```python
from build123d import *

# Parameters (mm, degrees)
SKETCH1_W               = 50.8
SKETCH1_H               = 25.4
BOSS_EXTRUDE1_DEPTH     = 3.999992
CUT_EXTRUDE1_DEPTH      = 57.936806514
CUT_EXTRUDE1_DEPTH_BACK = 57.936806514
SKETCH2_W               = 13.999972
SKETCH2_H               = 13.999972
SKETCH3_W               = 4.998974
SKETCH3_H               = 1.307084
CUT_EXTRUDE2_DEPTH      = 2.500122
BOSS_EXTRUDE2_DEPTH     = 50.8
FILLET1_R               = 1.5875


with BuildPart() as part:
    # Sketch1 → Boss-Extrude1 (new body)
    with BuildSketch(Plane(origin=(0, 0, 0), x_dir=(1, 0, 0), z_dir=(0, 1, 0))):
        with Locations((25.4, 12.7)):
            Rectangle(SKETCH1_W, SKETCH1_H)
    extrude(amount=BOSS_EXTRUDE1_DEPTH)

    # Sketch2 → Cut-Extrude1 (cut, two sides: drawn at the far end of the back side and taken through both)
    with BuildSketch(Plane(origin=(0, 3.999992, 0), x_dir=(1, 0, 0), z_dir=(0, 1, 0)).offset(-CUT_EXTRUDE1_DEPTH_BACK)):
        with Locations((15.875508, 12.7)):
            Rectangle(SKETCH2_W, SKETCH2_H)
        with Locations((34.924492, 12.7)):
            Rectangle(SKETCH2_W, SKETCH2_H)
    extrude(amount=CUT_EXTRUDE1_DEPTH + CUT_EXTRUDE1_DEPTH_BACK, mode=Mode.SUBTRACT)

    # Sketch3 → Cut-Extrude2 (cut)
    with BuildSketch(Plane(origin=(0, 3.999992, 0), x_dir=(1, 0, 0), z_dir=(0, 1, 0))):
        with Locations((15.875508, 20.353528)):
            Rectangle(SKETCH3_W, SKETCH3_H)
        with Locations((34.924492, 20.353528)):
            Rectangle(SKETCH3_W, SKETCH3_H)
        with Locations((34.924492, 5.046472)):
            Rectangle(SKETCH3_W, SKETCH3_H)
        with Locations((15.875508, 5.046472)):
            Rectangle(SKETCH3_W, SKETCH3_H)
    extrude(amount=-CUT_EXTRUDE2_DEPTH, mode=Mode.SUBTRACT)

    # Sketch5 → Boss-Extrude2 (add)
    with BuildSketch(Plane.ZY):
        Polygon((0, 0), (4.767004836, 3.999992), (0, 3.999992), align=None)
    extrude(amount=-BOSS_EXTRUDE2_DEPTH)

    # Fillet1
    fillet1_edges = [part.edges().sort_by_distance(p)[0] for p in [
        (25.4, 3.999992, 4.767004836),
    ]]
    fillet(fillet1_edges, radius=FILLET1_R)


solid = part.part
```
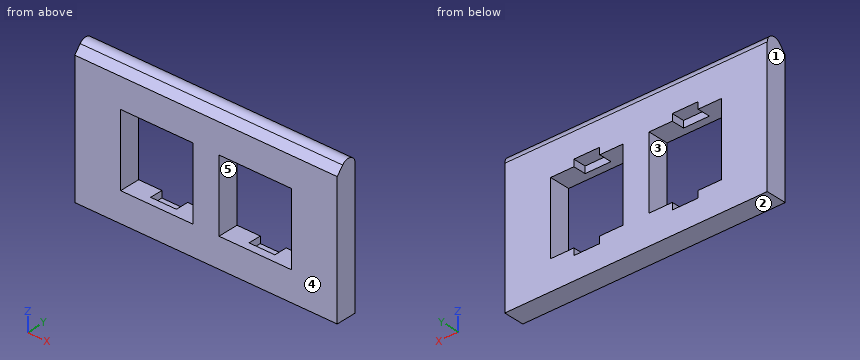
CAD build for the part. Positions are in the model's coordinates, mm. Face numbers are marked on the shaded views. A direction names the side the tool comes from. Coordinates: 2 decimals unless noted, no trailing zeros. Write each loop counter-clockwise with the first axis right and the second up, starting at its lowest first coordinate (ties: lowest second). Pieces come first, ordered by that corner, then holes. Notation, with made-up numbers: (52, 22.25) -> (101, 22.25) arc R23 ccw to (101, 57.25) -> close; hole circle Ø8 at (70.25, 56). An arc over 180 degrees is marked (long way). Return JSON: item names as keys, results as strings. Group by question number.
Q1. Drill centre lines: line 1 (X direction, y = 3.8, z = -8); line 2 (X direction, y = 3.05, z = -5) (3 decimals); line 3 (Z direction, x = 16.5, y = 1.4). Where is each one in solid material? Low to high.
Q2. Pull direction Z, two halves, no side cores. Call the marked faces 1, 2 and 3: released by +Z, released by -Z, zero draft, split by the parting line, or undercut.
Q3. Which spindle directions (+Z, -Z, +X, -X, +Y, -Y) get a long thin tool onto all of the face, cutting with end or side? Do the marked faces 4 and 5. Say none if no direction does.
Q4. Cut at D-D, the plane x = 7. Give the cut face in (y, z) (1 decimal).
Q5. Flat gauge pins, fed straight in: pin 1 (1 mm diameter, centred on y = 3.5, z = -5, fed in from -X); pin 2 (1 mm diameter, centred on x = 34.5, z = -20, fed in from +Y). Where does each tip first touch, or does it go through?
Q6. Cut at C-C, the plane y = 0.65. Give the cut face in (x, z).
Q7. Cut at B-B, the plane x = 19. Give the cut face in (y, z) (1 decimal), then the cut area to 3 significant figures.
Q8. Cut at A-A, the plane z = -14.75. Give the cut face in (x, y).
Returned:
{
 "1": {"line 1": "x = 0 to 8.88, 22.88 to 27.92, 41.92 to 50.8", "line 2": "x = 0 to 13.376, 18.375 to 32.425, 37.424 to 50.8", "line 3": "z = -25.4 to -19.7, -5.7 to 1.63"},
 "2": {"face 1": "zero draft", "face 2": "released by -Z", "face 3": "undercut"},
 "3": {"face 4": "+Z, -Z, +X, -X, -Y", "face 5": "+Y, -Y"},
 "4": {"outline": "(0, -25.4) -> (4, -25.4) -> (4, 0.4) arc R1.6 ccw to (1.2, 1.4) -> (0, 0) -> close"},
 "5": {"pin 1": "stops at x = 0", "pin 2": "stops at y = 1.5"},
 "6": {"outline": "(0, -25.4) -> (50.8, -25.4) -> (50.8, 0.77) -> (0, 0.77) -> close; hole (8.88, -19.7) -> (22.88, -19.7) -> (22.88, -5.7) -> (8.88, -5.7) -> close; hole (27.92, -19.7) -> (41.92, -19.7) -> (41.92, -5.7) -> (27.92, -5.7) -> close"},
 "7": {"outline": "(0, -25.4) -> (4, -25.4) -> (4, -19.7) -> (0, -19.7) -> close; (0, -5.7) -> (4, -5.7) -> (4, 0.4) arc R1.6 ccw to (1.2, 1.4) -> (0, 0) -> close", "area": "51.3 mm2"},
 "8": {"outline": "(0, 0) -> (8.88, 0) -> (8.88, 4) -> (0, 4) -> close; (22.88, 0) -> (27.92, 0) -> (27.92, 4) -> (22.88, 4) -> close; (41.92, 0) -> (50.8, 0) -> (50.8, 4) -> (41.92, 4) -> close"}
}
